```python
from build123d import *

# Parameters (mm, degrees)
SKETCH2_W               = 6.825797408
SKETCH2_H               = 2
CUT_EXTRUDE1_DEPTH      = 25
SKETCH3_R               = 1.5
BOSS_EXTRUDE1_DEPTH     = 2
SKETCH4_W               = 6.5
SKETCH4_H               = 10
BOSS_EXTRUDE2_DEPTH     = 24
SKETCH5_W               = 2.8
SKETCH5_H               = 6
CUT_EXTRUDE2_DEPTH      = 9
SKETCH6_R               = 1.55
CUT_EXTRUDE3_DEPTH      = 10
MIRROR4_COPY_1_SKETCH_R = 1.5
MIRROR4_COPY_1_DEPTH    = 2


with BuildPart() as part:
    # Sketch1 → Revolve1 (revolve)
    with BuildSketch(Plane.XY):
        Polygon((-2.660447761, -21.041604478), (-7.160447761, -21.041604478), (-7.160447761, 2.958395522), (-5.160447761, 2.958395522), (-5.160447761, -11.041604478), (-2.660447761, -11.041604478), align=None)
    revolve(axis=Axis((-0.110447761, 2.958395522, 0), (0, -1, 0)))

    # Sketch2 → Cut-Extrude1 (cut, through all)
    with BuildSketch(Plane(origin=(0, 2.958395522, 0), x_dir=(1, 0, 0), z_dir=(0, 1, 0))):
        with Locations((-5.160447761, 0)):
            Rectangle(SKETCH2_W, SKETCH2_H)
    extrude(amount=-CUT_EXTRUDE1_DEPTH, mode=Mode.SUBTRACT)

    # Sketch3 → Boss-Extrude1 (add)
    with BuildSketch(Plane.XY.offset(-1)):
        Polygon((-6.305854072, 1.958395522), (-11.305854072, -0.719474979), (-11.305854072, -5.719474979), (-6.305854072, -8.041604478), align=None)
        with Locations((-9.305854072, -3.157710953)):
            Circle(SKETCH3_R, mode=Mode.SUBTRACT)
    boss_extrude1 = extrude(amount=-BOSS_EXTRUDE1_DEPTH)

    # Mirror1: Boss-Extrude1 across plane
    add(boss_extrude1.mirror(Plane.XY))

    # Sketch4 → Boss-Extrude2 (add, through all)
    with BuildSketch(Plane(origin=(0, 2.958395522, 0), x_dir=(1, 0, 0), z_dir=(0, 1, 0))):
        with Locations((8.189552239, 0)):
            Rectangle(SKETCH4_W, SKETCH4_H)
    extrude(amount=-BOSS_EXTRUDE2_DEPTH)

    # Sketch5 → Cut-Extrude2 (cut)
    with BuildSketch(Plane(origin=(0, 2.958395522, 0), x_dir=(1, 0, 0), z_dir=(0, 1, 0))):
        with Locations((8.289552239, 0)):
            Rectangle(SKETCH5_W, SKETCH5_H)
    cut_extrude2 = extrude(amount=-CUT_EXTRUDE2_DEPTH, mode=Mode.SUBTRACT)

    # Mirror2: Cut-Extrude2 across plane
    add(cut_extrude2.mirror(Plane.ZX.offset(-9.041604478)), mode=Mode.SUBTRACT)

    # Sketch6 → Cut-Extrude3 (cut)
    with BuildSketch(Plane(origin=(11.439552239, 0, 0), x_dir=(0, 0, -1), z_dir=(1, 0, 0))):
        with Locations((-0.05, -3.291604478)):
            Circle(SKETCH6_R)
    cut_extrude3 = extrude(amount=-CUT_EXTRUDE3_DEPTH, mode=Mode.SUBTRACT)

    # Mirror3: Cut-Extrude3 across plane
    add(cut_extrude3.mirror(Plane.ZX.offset(-9.041604478)), mode=Mode.SUBTRACT)

    # Mirror4: Boss-Extrude1 across plane
    add(boss_extrude1.mirror(Plane.ZX.offset(-9.041604478)))

    # Mirror4 copy 1 sketch → Mirror4 copy 1 (add)
    with BuildSketch(Plane(origin=(0, -18.083208955, 1), x_dir=(1, 0, 0), z_dir=(0, 0, -1))):
        Polygon((-6.305854072, 1.958395522), (-11.305854072, -0.719474979), (-11.305854072, -5.719474979), (-6.305854072, -8.041604478), align=None)
        with Locations((-9.305854072, -3.157710953)):
            Circle(MIRROR4_COPY_1_SKETCH_R, mode=Mode.SUBTRACT)
    extrude(amount=-MIRROR4_COPY_1_DEPTH)


solid = part.part
```
Geometry check sheet. Reference: the model listing, model coordinates, mm. A direction names the side the tool comes from. Coordinates: 2 decimals unless noted, no trailing zeros. Write each loop counter-clockwise with the first axis right and the second up, starting at its lowest first coordinate (ties: lowest second). Pieces come first, ordered by that corner, then holes. Notation, with made-up numbers: M -37,74.25 L 3,74.25 A20 ccw 3,81.25 Z; hole C 1,7.5 d8. An arc over 180 degrees is marked long. Answer as a JSON object with one key per item and string values.
1. Scan lines: L1, parallel to Y at x = 10.8, z = 0.05; L2, parallel to Z at x = -8.75, y = -12; L3, parallel to Y at x = 3.75, z = 0.25. Record each from-to range of solid material in increasing order.
Answers below:
{"L1": "y = -21.04 to -16.34, -13.24 to -4.84, -1.74 to 2.96", "L2": "z = -3 to -1, 1 to 3", "L3": "y = -21.04 to -16.33, -13.25 to -11.04"}
2. Section check B-B, the plane y = -8.5. Enter the section's corners in (x, z).
Answers below:
{"outline": "M -7.09,-1 A7.05 ccw 4.94,-4.92 L 4.94,-5 L 11.44,-5 L 11.44,5 L 4.94,5 L 4.94,4.92 A7.05 ccw -7.09,1 L -5.06,1 A5.05 cw long -5.06,-1 Z"}
3. Draft check along Z on faces 1 (the flat face through (-7.9, -14, 3)), 2 (the cylindrical face through (-7.9, -14.4, -2)), 3 (the cylindrical face through (10.577, -1.755, 0.252)), 4 (the flat face through (6.89, -1, 0)). Enter one of: released by +Z, released by -Z, zero draft, split by the parting line, or undercut.
Answers below:
{"face 1": "released by +Z", "face 2": "zero draft", "face 3": "undercut", "face 4": "undercut"}
4. Tool access check on faces 5 (the flat face through (2, -11.042, 2)), 6 (the flat face through (-7.9, -14, -3)), 7 (the flat face through (9.69, -17, 0)). Record the directions out of +Z, -Z, +X, -X, +Y, -Y that give a thin tool (end or side, any length) a straight path to the whole face; none if there is none.
Answers below:
{"face 5": "+Y", "face 6": "-Z, -X, +Y, -Y", "face 7": "-Y"}
5. Go/stop test with flat-tipped pins: pin 1 Ø1.4 at (x, y) = (8, -18) entering from -Z; pin 2 Ø3 at (y, z) = (-3.29, 0.05) entering from +X; pin 3 Ø0.8 at (x, y) = (8, -17.5) entering from +Z; pin 4 Ø4 at (x, z) = (-0.11, 0) entering from -Y. Record where each tip stops, or that it passes through.
Answers below:
{"pin 1": "stops at z = -5", "pin 2": "stops at x = -4.92", "pin 3": "stops at z = 5", "pin 4": "passes through"}
6. Section check A-A, the plane x = -0.75. Enter the section's corners in (y, z).
Answers below:
{"outline": "M -21.04,-7.02 L 2.96,-7.02 L 2.96,-5.01 L -11.04,-5.01 L -11.04,-2.47 L -21.04,-2.47 Z; M -21.04,2.47 L -11.04,2.47 L -11.04,5.01 L 2.96,5.01 L 2.96,7.02 L -21.04,7.02 Z"}
7. Section check C-C, the plane z = 0.05. Give the number of separate pieces and of enclosed holes in the cut face, plus the area to 3 significant figures.
Answers below:
{"separate pieces": "5", "enclosed holes": "0", "area": "99.9 mm²"}
